Source: CAD feature listing. Evaluate the final solid. Frame: model axes, mm. A direction names the side the tool comes from. Give positions to 0.01 mm unless a question says otherwise; leave off trailing zeros. Order: outer loops, then holes, each group sorted by start corner. A loop starts at its lowest first (then second) coordinate and runs counter-clockwise, first axis right, second up. Notation, with made-up numbers: M 62,-4 L 98,-4 A20 cw 98,19 Z; hole C 59,37.5 d1. An arc over 180 degrees is marked long. Answer in a Markdown table with one row per item. Add a question column.
(1) Section query A-A, the plane x = 19.5. Return loops of the section in (y, z).
(2) Mould query, pull axis Y, two halves, no side actions, for faces 1 (the face through (76.92, 12.15, -30.53)), 2 (the face through (25, -4, 8)), 3 (the face through (70.26, -0.92, -22.78)), 4 (the face through (57.52, 0.434, -7.593)). Classes: pulls with the +Y half, pulls with the -Y half, needs draft (parallel to the pull), parting line crosses it, or undercut.
(3) Set-up query: faces 5 (the face through (43, 15, 2)), 6 (the face through (23, -4, 0)), 7 (the face through (32.73, -0.07, 3.94)). Return all of +Z, -Z, +X, -X, +Y, -Y with unobstructed straight access to the full face (end or side cutting, diameter ignored); none if empty.
(4) Section query B-B, the plane y = 0. Return loops of the section in (x, z), plus the area to 3 significant figures.
(5) Pin query (flat end, axial travel): P1, Ø9, axis at x = 11.5, y = -1, coming from the -Z side; P2, Ø6, axis at y = 9.5, z = -24.5, coming from the -X side. Return the tip coordinate at first contact, or that it passes through.
(6) Section query C-C, the plane x = 44. Return loops of the section in (y, z), plus the area to 3 significant figures.
(7) Section query D-D, the plane y = -6. Return loops of the section in (x, z), plus the area to 3 significant figures.
(8) Material intervals for line 1 along Y through (x, z) = (29, 0.5); line 2 along Z through (x, y) = (34.5, 3.5); line 3 along X through (y, z) = (-8, -19), sorted ascending.
from build123d import *

# Parameters (mm, degrees)
F1_DEPTH = 15
F3_DEPTH = 8.001
F5_D     = 4
F6_R     = 10
F7_SIZE  = 5


with BuildPart() as f1:
    # F0 (on Front) → F1 (new body, symmetric)
    with BuildSketch(Plane.XZ):
        Polygon((0, 0), (46, 0), (75.7414862046, -35.4445230334), (81.8698417496, -30.3022221559), (49.7304612652, 8), (-0.2695387348, 8), align=None)
    extrude(amount=F1_DEPTH, both=True)

    # F2 (on Top) → F3 (cut, through all)
    with BuildSketch(Plane.XY):
        with BuildLine():
            ThreePointArc((14.7304612652, 3), (11.7304612652, 0), (14.7304612652, -3))
            Line((14.7304612652, -3), (29.7304612652, -3))
            ThreePointArc((29.7304612652, -3), (32.7304612652, 0), (29.7304612652, 3))
            Line((29.7304612652, 3), (14.7304612652, 3))
        make_face()
    extrude(amount=F3_DEPTH, mode=Mode.SUBTRACT)

    # F5 (through all)
    with Locations(Plane(origin=(33.1222636313, 0, 27.7928791968), x_dir=(0, 1, 0), z_dir=(0.7660444431, 0, 0.6427876097))):
        with Locations((0, -40.8377687803), (0, -60.8377687803)):
            Hole(F5_D / 2)

    # F6
    f6_edges = [f1.edges().sort_by_distance(p)[0] for p in [
        (78.805664, -15, -32.873373),
        (78.805664, 15, -32.873373),
    ]]
    fillet(f6_edges, radius=F6_R)

    # F7
    f7_edges = [f1.edges().sort_by_distance(p)[0] for p in [
        (-0.134769, 15, 4),
        (-0.134769, -15, 4),
    ]]
    chamfer(f7_edges, length=F7_SIZE)


solid = f1.part
Values follow:
| question | item | result |
|---|---|---|
| 1 | outline | M -15,0 L -3,0 L -3,8 L -15,8 Z; M 3,0 L 15,0 L 15,8 L 3,8 Z |
| 2 | face 1 | pulls with the +Y half |
| 2 | face 2 | needs draft |
| 2 | face 3 | undercut |
| 2 | face 4 | undercut |
| 3 | face 5 | +Z, -Z, +X, -X, +Y |
| 3 | face 6 | -Z, -X, +Y, -Y |
| 3 | face 7 | +Z, -Z |
| 4 | outline | M -0.27,8 L 0,0 L 11.73,0 L 11.73,8 Z; M 32.73,0 L 46,0 L 51.96,-7.1 L 58.09,-1.96 L 49.73,8 L 32.73,8 Z; M 54.53,-10.17 L 64.81,-22.42 L 70.94,-17.28 L 60.66,-5.02 Z; M 67.39,-25.49 L 75.74,-35.44 L 81.87,-30.3 L 73.51,-20.34 Z |
| 4 | area | 537 mm² |
| 5 | P1 | stops at z = 0 |
| 5 | P2 | stops at x = 64.04 |
| 6 | outline | M -15,0 L 15,0 L 15,8 L -15,8 Z |
| 6 | area | 240 mm² |
| 7 | outline | M -0.27,8 L 0,0 L 46,0 L 75.71,-35.41 L 81.84,-30.26 L 49.73,8 Z |
| 7 | area | 769 mm² |
| 8 | line 1 | y = -15 to -3, 3 to 15 |
| 8 | line 2 | z = 0 to 8 |
| 8 | line 3 | x = 61.94 to 72.39 |
